Answer from the drawing. Dimensions are ordinates in mm from the lowest x, y and z of the part. A direction names the side the tool comes from. Coordinates: 2 decimals unless noted, no trailing zeros. Order: outer loops, then holes, each group sorted by start corner. A loop starts at its lowest first (then second) coordinate and runs counter-clockwise, first axis right, second up. Notation, with made-up numbers: (47.5, -13) - (59.5, -13) arc R20 ccw to (59.5, 12) - close; hole circle Ø4 at (57, 83.25). An arc over 180 degrees is marked (long way). Answer as a JSON object with one key per item and string values. Group by question number.
1) Section C-C (y = 32) is taken. Give the vertices of the cut face in (x, z).
2) A tool of negligible diameter and unlimited length cuts with its end or side. For the marked faces 1, 2, 3 and 4, from which of +Z, -Z, +X, -X, +Y, -Y can it reach the whole face along a straight path? Write none if from no direction.
3) Section A-A (z = 7.75) is taken. Give the vertices of the cut face in (x, y).
4) Each of these flat-tipped pins is pushed along its axis until it touches: P1, Ø0.6, axis at x = 10.5, y = 2, coming from the -Z side; P2, Ø2, axis at y = 3.5, z = 7.5, coming from the -X side; P3, Ø6, axis at y = 23.5, z = 7, coming from the -X side; P4, Ø3, axis at y = 4, z = 3, coming from the -X side. Where does it stop, or does it pass through?
5) Find the intervals of material crossed by line 1 along X through (y, z) = (5, 6.5); line 2 along Y through (x, z) = (2.75, 11.25); line 3 along Y through (x, z) = (3, 1.25), in increasing order.
6) Section B-B (x = 7.75) is taken. Give the vertices of the cut face in (y, z), plus the area to 3 significant figures.
7) Section D-D (y = 21) is taken. Give the vertices of the cut face in (x, z).
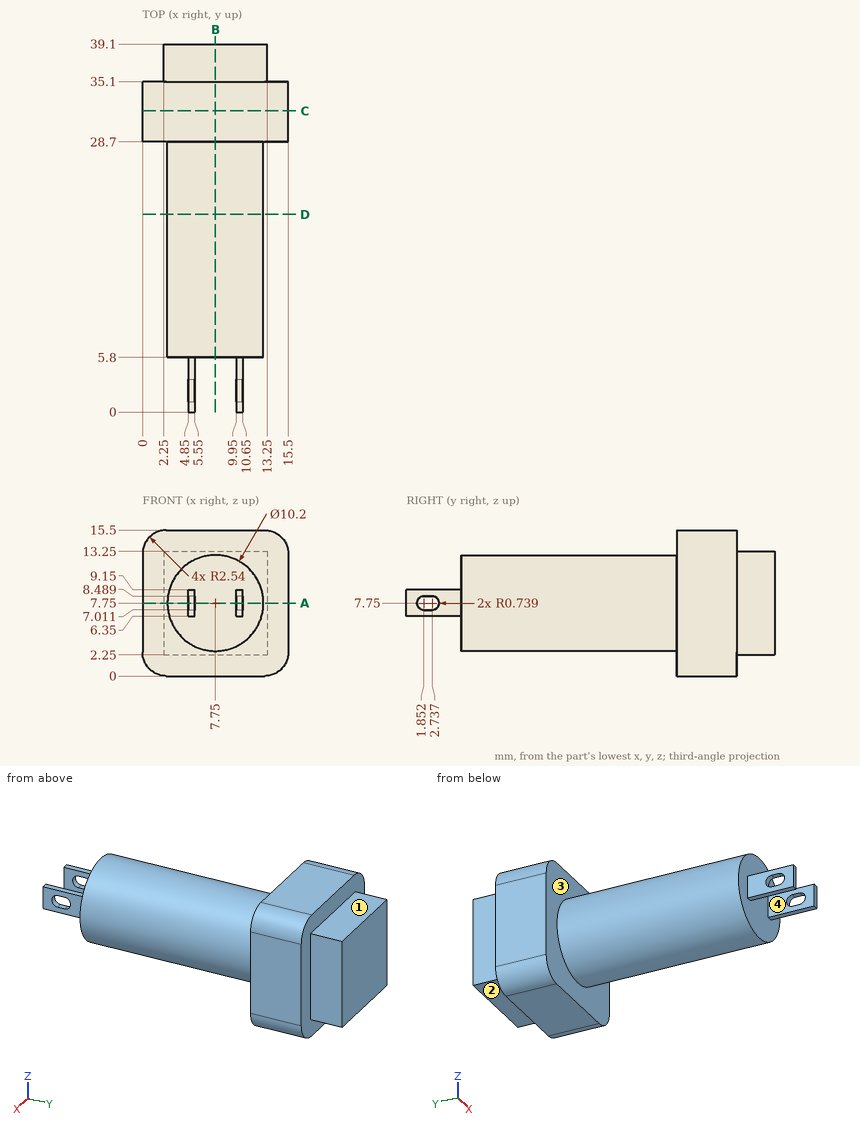
Report:
{
 "1": {"outline": "(0, 2.54) arc R2.54 ccw to (2.54, 0) - (12.96, 0) arc R2.54 ccw to (15.5, 2.54) - (15.5, 12.96) arc R2.54 ccw to (12.96, 15.5) - (2.54, 15.5) arc R2.54 ccw to (0, 12.96) - close"},
 "2": {"face 1": "+Z, +X, -X, +Y", "face 2": "-Z, +X, -X, +Y", "face 3": "-Y", "face 4": "+Z, -Z, -Y"},
 "3": {"outline": "(0, 28.7) - (2.65, 28.7) - (2.65, 5.8) - (4.85, 5.8) - (4.85, 3.48) - (5.55, 3.48) - (5.55, 5.8) - (9.95, 5.8) - (9.95, 3.48) - (10.65, 3.48) - (10.65, 5.8) - (12.85, 5.8) - (12.85, 28.7) - (15.5, 28.7) - (15.5, 35.1) - (13.25, 35.1) - (13.25, 39.1) - (2.25, 39.1) - (2.25, 35.1) - (0, 35.1) - close; (4.85, 0) - (5.55, 0) - (5.55, 1.11) - (4.85, 1.11) - close; (9.95, 0) - (10.65, 0) - (10.65, 1.11) - (9.95, 1.11) - close"},
 "4": {"P1": "stops at z = 6.35", "P2": "stops at x = 4.85", "P3": "stops at x = 2.65", "P4": "passes through"},
 "5": {"line 1": "x = 4.85 to 5.55, 9.95 to 10.65", "line 2": "y = 28.7 to 39.1", "line 3": "y = 28.7 to 35.1"},
 "6": {"outline": "(5.8, 2.65) - (28.7, 2.65) - (28.7, 0) - (35.1, 0) - (35.1, 2.25) - (39.1, 2.25) - (39.1, 13.25) - (35.1, 13.25) - (35.1, 15.5) - (28.7, 15.5) - (28.7, 12.85) - (5.8, 12.85) - close", "area": "377 mm²"},
 "7": {"outline": "circle Ø10.2 at (7.75, 7.75)"}
}
